Could you check a few things on this model? Use its own coordinates, in mm. Face numbers are marked on the shaded views. A direction names the side the tool comes from. Coordinates: 2 decimals unless noted, no trailing zeros. Order: outer loops, then holes, each group sorted by start corner. A loop starts at its lowest first (then second) coordinate and runs counter-clockwise, first axis right, second up.
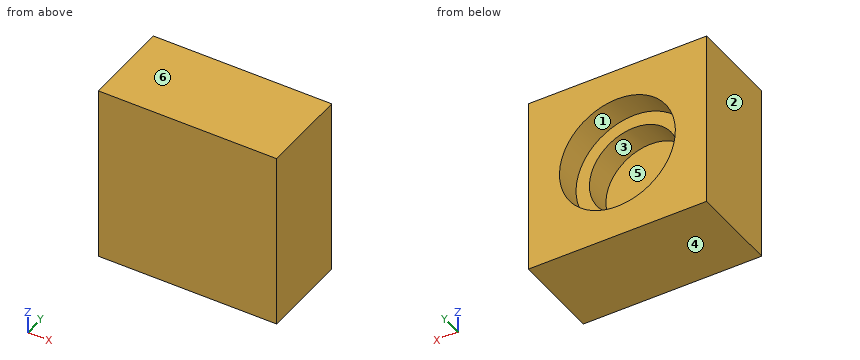
```python
from build123d import *

# Parameters (mm, degrees)
SKETCH_1_W          = 40
SKETCH_1_H          = 40
EXTRUDE_1_DEPTH     = 20
SKETCH_2_R          = 13
CUT_EXTRUDE_1_DEPTH = 6
SKETCH_3_R          = 10
CUT_EXTRUDE_2_DEPTH = 6


with BuildPart() as part:
    # Эскиз1 → Бобышка-Вытянуть1 (new body)
    with BuildSketch(Plane(origin=(0, 0, 0), x_dir=(1, 0, 0), z_dir=(0, 1, 0))):
        with Locations((20, 20)):
            Rectangle(SKETCH_1_W, SKETCH_1_H)
    extrude(amount=EXTRUDE_1_DEPTH)

    # Эскиз2 → Вырез-Вытянуть1 (cut)
    with BuildSketch(Plane(origin=(0, 20, 0), x_dir=(1, 0, 0), z_dir=(0, 1, 0))):
        with Locations(Location((20, 20, 0), (0, 0, 270))):
            Circle(SKETCH_2_R)
    extrude(amount=-CUT_EXTRUDE_1_DEPTH, mode=Mode.SUBTRACT)

    # Эскиз3 → Вырез-Вытянуть2 (cut)
    with BuildSketch(Plane(origin=(0, 14, 0), x_dir=(1, 0, 0), z_dir=(0, 1, 0))):
        with Locations(Location((20, 20, 0), (0, 0, 270))):
            Circle(SKETCH_3_R)
    extrude(amount=-CUT_EXTRUDE_2_DEPTH, mode=Mode.SUBTRACT)


solid = part.part
```
Item 1: For pin 1 Ø6 at (x, z) = (22.5, -20.5) entering from +Y, with a flat end and sliding along its axis, tell me the tip position at first contact or that it passes through.
Item 2: Suppose I cut it at B-B (z = -20). List the corners of the cut face in (x, y) for me, and give its area (3 significant figures).
Item 3: Suppose I cut it at D-D (x = 8). List the corners of the cut face in (y, z) for me, and give its area (3 significant figures).
Item 4: Which directions (+Z, -Z, +X, -X, +Y, -Y) give clear straight access to the entire face, cutting with the end or side of a thin tool? Please do the marked faces 5 and 6.
Item 5: I need wall thicknesses on line 1 (X direction, y = 18.7, z = -20); line 2 (X direction, y = 10.7, z = -20); line 3 (Y direction, x = 28.5, z = -29). Which ranges of each line are inside material? Lowest first, please.
Item 6: Suppose I cut it at C-C (x = 20). List the corners of the cut face in (y, z) for me, and give its area (3 significant figures).
Item 7: Thinking about a two-plate mould opening in X: for the marked faces 1, 2, 3 and 4, which applies, +X half, -X half, draft (parallel to the pull), parting line (faces both ways), or undercut?
Item 8: Suppose I cut it at A-A (y = 12.25). List the corners of the cut face in (x, z) for me.
Geometry results:
1. pin 1: stops at y = 8
2. outline: (0, 0) - (40, 0) - (40, 20) - (33, 20) - (33, 14) - (30, 14) - (30, 8) - (10, 8) - (10, 14) - (7, 14) - (7, 20) - (0, 20) - close
2. area: 524 mm2
3. outline: (0, -40) - (20, -40) - (20, -25) - (14, -25) - (14, -15) - (20, -15) - (20, 0) - (0, 0) - close
3. area: 740 mm2
4. face 5: +Y
4. face 6: +Z, +X, -X, +Y, -Y
5. line 1: x = 0 to 7, 33 to 40
5. line 2: x = 0 to 10, 30 to 40
5. line 3: y = 0 to 14
6. outline: (0, -40) - (20, -40) - (20, -33) - (14, -33) - (14, -30) - (8, -30) - (8, -10) - (14, -10) - (14, -7) - (20, -7) - (20, 0) - (0, 0) - close
6. area: 524 mm2
7. face 1: undercut
7. face 2: -X half
7. face 3: undercut
7. face 4: draft
8. outline: (0, -40) - (40, -40) - (40, 0) - (0, 0) - close; hole circle Ø20 at (20, -20)
